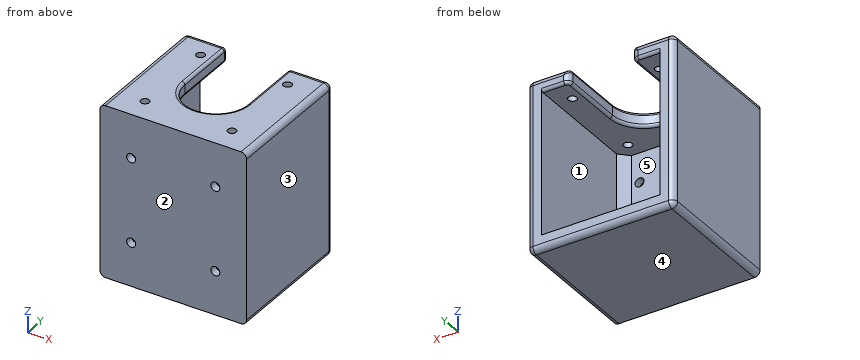
Autodesk Inventor part; units mm, degrees
sketch "Эскиз1" plane through (0, 0, 0) normal (0, 1, 0) x (-1, 0, 0)
  line L0 (21.15, 25.5) -> (-21.15, 25.5)
  line L1 (-21.15, 25.5) -> (-21.15, -25.5)
  line L2 (-21.15, -25.5) -> (21.15, -25.5)
  line L3 (21.15, -25.5) -> (21.15, 25.5)
  line L4 (21.15, 25.5) -> (-21.15, -25.5) construction
  line L5 (-21.15, 25.5) -> (21.15, -25.5) construction
  point P0 (0, 0)
  dimension "d2" = 51
  dimension "d3" = 42.3
extrude "Выдавливание1" add sketch "Эскиз1" along normal mid plane 2.85
sketch "Эскиз2" plane through (0, 1.425, 0) normal (0, 1, 0) x (1, 0, 0)
  line L0 (-21.15, -25.5) -> (-21.15, 25.5)
  line L1 (-21.15, 25.5) -> (-26.15, 25.5)
  line L2 (-26.15, 25.5) -> (-26.15, -25.5)
  line L3 (-26.15, -25.5) -> (-21.15, -25.5)
  line L4 (-21.15, -25.5) -> (-21.15, 25.5)
  point P0 (0, 0)
  dimension "d4" = 5
extrude "Выдавливание2" add sketch "Эскиз2" along normal blind 45.15 and the other way blind 2.85
mirror "Зеркальное отражение1" about plane through (0, 0, 0) normal (1, 0, 0) of "Выдавливание2"
chamfer "Фаска1" distance 3.2 angle 45 2 edges at (-21.15, 1.425, 0) (21.15, 1.425, 0)
sketch "Эскиз3" plane through (0, 1.425, 0) normal (0, 1, 0) x (1, 0, 0)
  line L0 (-26.15, 25.5) -> (26.15, 25.5)
  line L1 (-26.15, 25.5) -> (26.15, 25.5)
  line L2 (26.15, 25.5) -> (26.15, 30.5)
  line L3 (26.15, 30.5) -> (-26.15, 30.5)
  line L4 (-26.15, 30.5) -> (-26.15, 25.5)
  point P0 (0, 0)
  dimension "d17" = 5
extrude "Выдавливание3" add sketch "Эскиз3" along normal blind 45.15 and the other way blind 2.85
mirror "Зеркальное отражение2" about plane through (0, 0, 0) normal (0, 0, 1) of "Выдавливание3"
sketch "Эскиз7" plane through (-26.15, -1.425, 30.5) normal (0, 0, 1) x (1, 0, 0)
  circle A0 centre (26.15, 24) radius 11
  circle A1 centre (26.15, 24) radius 11.2
  point P0 (26.15, 1.425)
  dimension "d22" = 22.4
extrude "Выдавливание5" cut sketch "Эскиз7" against normal up to next contours A0 | A1
sketch "Эскиз8" plane through (-26.15, -1.425, 30.5) normal (0, 0, 1) x (1, 0, 0)
  circle A0 centre (26.15, 24) radius 11.2
  line L0 (14.95, 24) -> (14.95, 48)
  line L1 (5, 48) -> (47.3, 48)
  line L2 (37.35, 24) -> (37.35, 48.1316)
  point P0 (26.15, 1.425)
  point P1 (37.35, 48)
  dimension "d23" = 22.4
extrude "Выдавливание6" cut sketch "Эскиз8" against normal up to next contours A0 L0 L1 L2
fillet "Сопряжение1" radius 2 11 edges at (-11.2, 46.575, 28) (11.2, 46.575, 28) (-26.15, 46.575, 0) (-18.675, 46.575, 30.5) (18.675, 46.575, 30.5) (26.15, 46.575, 0) (0, 46.575, -30.5) (26.15, 22.575, 30.5) (-26.15, 22.575, 30.5) (-26.15, 22.575, -30.5) (26.15, 22.575, -30.5)
fillet "Сопряжение2" radius 1 12 edges at (0, 11.375, 25.5) (11.2, 33.575, 25.5) (11.7858, 45.9892, 25.5) (17.175, 46.575, 25.5) (-11.7858, 45.9892, 25.5) (-17.175, 46.575, 25.5) (-11.2, 33.575, 25.5) (-11.7858, 45.9892, 29.9142) (0, 11.375, 30.5) (11.2, 33.575, 30.5) (11.7858, 45.9892, 29.9142) (-11.2, 33.575, 30.5)
sketch "Эскиз9" plane through (-24.15, -1.425, 30.5) normal (0, 0, 1) x (1, 0, 0)
  circle A0 centre (8.65, 39.5) radius 1.5
  circle A1 centre (39.65, 39.5) radius 1.5
  circle A2 centre (39.65, 8.5) radius 1.5
  circle A3 centre (8.65, 8.5) radius 1.5
  line L0 (8.65, 39.5) -> (39.65, 39.5) construction
  line L1 (39.65, 39.5) -> (39.65, 8.5) construction
  line L2 (39.65, 8.5) -> (8.65, 8.5) construction
  line L3 (8.65, 8.5) -> (8.65, 39.5) construction
  arc A4 (12.95, 24) -> (35.35, 24) centre (24.15, 24) ccw
  line L4 (8.65, 39.5) -> (39.65, 8.5) construction
  line L5 (39.65, 39.5) -> (8.65, 8.5) construction
  line L6 (24.15, 62.1506) -> (24.15, -10.3584)
  point P0 (24.15, 1.425)
  point P1 (24.15, 24)
  point P2 (24.15, 24)
  dimension "d28" = 3
  dimension "d29" = 31
extrude "Выдавливание7" cut sketch "Эскиз9" against normal up to next
sketch "Эскиз10" plane through (0, -1.425, 0) normal (0, -1, 0) x (1, 0, 0)
  line L0 (15, -15) -> (-15, -15) construction
  line L1 (-15, -15) -> (-15, 15) construction
  line L2 (-15, 15) -> (15, 15) construction
  line L3 (15, 15) -> (15, -15) construction
  line L4 (15, -15) -> (-15, 15) construction
  line L5 (-15, -15) -> (15, 15) construction
  circle A0 centre (-15, -15) radius 1.6
  circle A1 centre (-15, 15) radius 1.6
  circle A2 centre (15, -15) radius 1.6
  circle A3 centre (15, 15) radius 1.6
  point P0 (0, 0)
  dimension "d32" = 30
  dimension "d33" = 3.2
extrude "Выдавливание8" cut sketch "Эскиз10" against normal up to next
properties part number "Крепление_мотора"
Source: CAD feature listing. Evaluate the final solid. Frame: model axes, mm. Face numbers are marked on the shaded views. A direction names the side the tool comes from. Give positions to 0.01 mm unless a question says otherwise; leave off trailing zeros. Write each loop counter-clockwise with the first axis right and the second up, starting at its lowest first coordinate (ties: lowest second). Pieces come first, ordered by that corner, then holes.
1. Pull-direction query (Z, two-part tool) for the marked faces 3, 4 and 5; classes: +Z half, -Z half, draft (parallel to the pull), parting line (faces both ways), or undercut.
2. Material intervals for line 1 along Y through (x, z) = (15.5, 26.85) (3 decimals); line 2 along Z through (x, y) = (15, 0); line 3 along X through (y, z) = (18.5, 25), sorted ascending.
3. Section query B-B (y = 24.5). Return the cut outline in (x, z).
4. Section query D-D (x = 0). Return the cut outline in (y, z) (3 decimals), then the cut area to 3 significant figures.
5. First-contact query: pin 1 (3.5 mm diameter, centred on x = -15, z = -15, fed in from -Y) (3 decimals); pin 2 (1.9 mm diameter, centred on x = 15, z = 15, fed in from -Y); pin 3 (10 mm diameter, centred on x = 6.5, z = 0.5, fed in from +Y) (3 decimals); pin 4 (12.5 mm diameter, centred on x = 3.5, y = 18.5, fed in from +Z). Flat tips, straight axial feed; report the tip coordinate or a pass-through.
6. Section query A-A (z = 15). Return the cut outline in (x, y) (3 decimals).
7. Access query for the marked faces 1 and 2. Directions: +Z, -Z, +X, -X, +Y, -Y. A direction counts if a zero-diameter tool reaches every point of the face in a straight line with its end or side. Return the directions, or none.
8. Section query C-C (x = -15). Return the cut outline in (y, z) (3 decimals), then the cut area to 3 significant figures.
Output values:
1. face 3: draft
1. face 4: -Z half
1. face 5: undercut
2. line 1: y = -1.425 to 5.575, 8.575 to 36.575, 39.575 to 46.575
2. line 2: z = -30.5 to -16.6, -13.4 to 13.4, 16.6 to 30.5
2. line 3: x = -26.15 to -21.15, 21.15 to 26.15
3. outline: (-26.15, -28.5) arc R2 ccw to (-24.15, -30.5) - (24.15, -30.5) arc R2 ccw to (26.15, -28.5) - (26.15, 28.5) arc R2 ccw to (24.15, 30.5) - (12.2, 30.5) arc R1 ccw to (11.2, 29.5) - (11.2, 26.5) arc R1 ccw to (12.2, 25.5) - (21.15, 25.5) - (21.15, -25.5) - (-21.15, -25.5) - (-21.15, 25.5) - (-12.2, 25.5) arc R1 ccw to (-11.2, 26.5) - (-11.2, 29.5) arc R1 ccw to (-12.2, 30.5) - (-24.15, 30.5) arc R2 ccw to (-26.15, 28.5) - close
4. outline: (-1.425, -30.5) - (44.575, -30.5) arc R2 ccw to (46.575, -28.5) - (46.575, -25.5) - (1.425, -25.5) - (1.425, 25.5) - (10.375, 25.5) arc R1 ccw to (11.375, 26.5) - (11.375, 29.5) arc R1 ccw to (10.375, 30.5) - (-1.425, 30.5) - close
4. area: 448 mm2
5. pin 1: stops at y = -1.425
5. pin 2: passes through
5. pin 3: stops at y = 1.425
5. pin 4: stops at z = 30.32
6. outline: (-26.15, -1.425) - (-16.6, -1.425) - (-16.6, 1.425) - (-17.95, 1.425) - (-21.15, 4.625) - (-21.15, 46.575) - (-24.15, 46.575) arc R2 ccw to (-26.15, 44.575) - close; (-13.4, -1.425) - (13.4, -1.425) - (13.4, 1.425) - (-13.4, 1.425) - close; (16.6, -1.425) - (26.15, -1.425) - (26.15, 44.575) arc R2 ccw to (24.15, 46.575) - (21.15, 46.575) - (21.15, 4.625) - (17.95, 1.425) - (16.6, 1.425) - close
7. face 1: +Y
7. face 2: +Z, -Z, +X, -X, -Y
8. outline: (-1.425, -30.5) - (44.575, -30.5) arc R2 ccw to (46.575, -28.5) - (46.575, -25.5) - (1.425, -25.5) - (1.425, -16.6) - (-1.425, -16.6) - close; (-1.425, -13.4) - (1.425, -13.4) - (1.425, 13.4) - (-1.425, 13.4) - close; (-1.425, 16.6) - (1.425, 16.6) - (1.425, 25.5) - (5.661, 25.5) - (5.661, 30.5) - (-1.425, 30.5) - close; (8.489, 25.5) - (36.661, 25.5) - (36.661, 30.5) - (8.489, 30.5) - close; (39.489, 25.5) - (45.575, 25.5) arc R1 ccw to (46.575, 26.5) - (46.575, 28.5) arc R2 ccw to (44.575, 30.5) - (39.489, 30.5) - close
8. area: 577 mm2
